Input: part model. Units: mm. Frame: model coordinates. Coordinates: 2 decimals unless noted, no trailing zeros. Loops run counter-clockwise (first coordinate to the right, second up) from the corner with the lowest first, then second, coordinate; pieces in that order, holes last. Notation, with made-up numbers: (34, 70.25) - (45, 70.25) arc R20 ccw to (45, 106.25) - close; hole circle Ø5 at (27.5, -14). An arc over 180 degrees is marked (long way). Write item = value, one per line. Start each with the question number.
from build123d import *

# Parameters (mm, degrees)
F0_W     = 203.2
F0_H     = 38.1
F1_DEPTH = 3.175
F2_W     = 3.175
F2_H     = 4.445
F3_DEPTH = 25.4


# Not quite as in the source:
# - a feature names something its author has since deleted; it is built from what else it names


with BuildPart() as f1:
    # F0 (on Top) → F1 (new body)
    with BuildSketch(Plane.XY):
        with Locations((101.6, -19.05)):
            Rectangle(F0_W, F0_H)
    extrude(amount=F1_DEPTH)

    # F2 (on face) → F3 (cut)
    with BuildSketch(Plane.XY.offset(3.175)):
        with BuildLine():
            Line((0, -9.525), (0, -14.2875))
            ThreePointArc((0, -14.2875), (24.649723028, -4.4760985439), (50.8, 0))
            Line((50.8, 0), (0, 0))
            Line((0, 0), (0, -9.525))
        make_face()
        with Locations((103.1875, -35.8775)):
            Rectangle(F2_W, F2_H)
        with BuildLine():
            ThreePointArc((104.775, -30.48), (103.8450640303, -32.7250640303), (101.6, -33.655))
            Line((101.6, -33.655), (104.775, -33.655))
            Line((104.775, -33.655), (104.775, -30.48))
        make_face()
        with BuildLine():
            Line((104.775, -30.48), (101.6, -30.48))
            Line((101.6, -30.48), (101.6, -33.655))
            ThreePointArc((101.6, -33.655), (103.8450640303, -32.7250640303), (104.775, -30.48))
        make_face()
        with BuildLine():
            Line((101.6, -27.305), (101.6, -30.48))
            Line((101.6, -30.48), (104.775, -30.48))
            ThreePointArc((104.775, -30.48), (103.8450640303, -28.2349359697), (101.6, -27.305))
        make_face()
        with BuildLine():
            Line((98.4250000029, -30.4801362911), (101.6, -30.48))
            Line((101.6, -30.48), (101.6, -27.305))
            ThreePointArc((101.6, -27.305), (99.3548877841, -28.2349841564), (98.4250000029, -30.4801362911))
        make_face()
        with BuildLine():
            Line((101.6, -33.655), (101.6, -30.48))
            Line((101.6, -30.48), (98.4250000029, -30.4801362911))
            ThreePointArc((98.4250000029, -30.4801362911), (99.3549841564, -32.7251122159), (101.6, -33.655))
        make_face()
        with BuildLine():
            ThreePointArc((108.3690122037, -30.48), (106.4969075417, -31.9824905065), (104.775, -33.655))
            Line((104.775, -33.655), (104.775, -38.1))
            Line((104.775, -38.1), (184.15, -38.1))
            Line((184.15, -38.1), (193.675, -26.19375))
            ThreePointArc((193.675, -26.19375), (163.9135585822, -23.6655567526), (134.3847364187, -28.1581971794))
            ThreePointArc((134.3847364187, -28.1581971794), (121.0555708247, -25.7189035938), (108.3690122037, -30.48))
        make_face()
        with BuildLine():
            Line((101.6, -38.1), (101.6, -33.655))
            ThreePointArc((101.6, -33.655), (99.3549841564, -32.7251122159), (98.4250000029, -30.4801362911))
            Line((98.4250000029, -30.4801362911), (39.6036359929, -30.4826612755))
            ThreePointArc((39.6036359929, -30.4826612755), (18.2099329026, -26.2778753266), (0, -14.2875))
            Line((0, -14.2875), (0, -19.05))
            Line((0, -19.05), (0, -38.1))
            Line((0, -38.1), (101.6, -38.1))
        make_face()
        Polygon((203.2, 0), (184.15, 0), (203.2, -14.2875), align=None)
        Polygon((193.675, -26.19375), (184.15, -38.1), (203.2, -38.1), (203.2, -19.05), (203.2, -14.2875), align=None)
        with BuildLine():
            Line((108.3690122037, -30.48), (104.775, -30.48))
            Line((104.775, -30.48), (104.775, -33.655))
            ThreePointArc((104.775, -33.655), (106.4969075417, -31.9824905065), (108.3690122037, -30.48))
        make_face()
        with BuildLine():
            ThreePointArc((127.6218066335, -14.2875), (122.8593066335, -9.525), (118.0968066335, -14.2875))
            Line((118.0968066335, -14.2875), (127.6218066335, -14.2875))
        make_face()
        with BuildLine():
            Line((127.6218066335, -14.2875), (118.0968066335, -14.2875))
            ThreePointArc((118.0968066335, -14.2875), (122.8593066335, -19.05), (127.6218066335, -14.2875))
        make_face()
        with BuildLine():
            Line((176.8343066335, -14.2875), (183.1843066335, -14.2875))
            ThreePointArc((183.1843066335, -14.2875), (180.0093066335, -11.1125), (176.8343066335, -14.2875))
        make_face()
        with BuildLine():
            ThreePointArc((176.8343066335, -14.2875), (180.0093066335, -17.4625), (183.1843066335, -14.2875))
            Line((183.1843066335, -14.2875), (176.8343066335, -14.2875))
        make_face()
        with BuildLine():
            ThreePointArc((155.4030566335, -14.2875), (151.4343066335, -10.31875), (147.4655566335, -14.2875))
            Line((147.4655566335, -14.2875), (155.4030566335, -14.2875))
        make_face()
        with BuildLine():
            Line((155.4030566335, -14.2875), (147.4655566335, -14.2875))
            ThreePointArc((147.4655566335, -14.2875), (151.4343066335, -18.25625), (155.4030566335, -14.2875))
        make_face()
    extrude(amount=-F3_DEPTH, mode=Mode.SUBTRACT)

    # F8: sweep along a path in F5
    with BuildLine(Plane.XY.offset(1.5875)) as f8_path:
        Line((101.6, -30.48), (39.6036359929, -30.4826612755))
        ThreePointArc((39.6036359929, -30.4826612755), (18.2099329026, -26.2778753266), (0, -14.2875))
    # F7 (on offset) → F8 (sweep, cut)
    with BuildSketch(Plane.YZ.offset(101.6)):
        Polygon((-30.48, 3.1877), (-30.48, 1.5875), (-4.1187478461, 6.2357), (-30.48, 6.2357), align=None)
        Polygon((-30.48, 1.5875), (-30.48, 0), (-30.48, -3.0607), (-4.1187478461, -3.0607), align=None)
    sweep(path=f8_path.line, mode=Mode.SUBTRACT)


solid = f1.part
Item 1: Ray query, line 1 (Y direction, x = 123, z = 1.7); line 2 (X direction, y = -12, z = 2.4); line 3 (Y direction, x = 181, z = 0.8). Return the intervals inside material, ascending.
Item 2: Cut plane C-C on x = 90. Return loops of the section in (y, z) (1 decimal).
Item 3: Cut plane B-B on z = 0.5. State how many separate pieces and enclosed holes the cut face has, plus the area to 3 significant figures.
Item 4: Pull-direction query (X, two-part tool) for faces 1 (the flat face through (198.5, -20.16, 1.61)), 2 (the cylindrical face through (24.292, -4.577, 1.61)), 3 (the cylindrical face through (118.317, -15.718, 1.61)); classes: pulls with the +X half, pulls with the -X half, needs draft (parallel to the pull), parting line crosses it, or undercut.
Item 5: Cut plane A-A on x = 46.5. Return loops of the section in (y, z) (1 decimal).
Item 6: Pin query (flat end, axial travel): pin 1 (1 mm diameter, centred on x = 106.5, z = 2, fed in from -Y); pin 2 (1.5 mm diameter, centred on y = -6.5, z = 1, fed in from +X). Return the tip coordinate at first contact, or that it passes through.
Item 7: Cut plane D-D on x = 139. Return loops of the section in (y, z) (3 decimals).
Recorded:
q1.line_1 = -25.62 to -19.05, -9.53 to 0
q1.line_2 = 4.58 to 118.68, 127.04 to 148.19, 154.68 to 177.81, 182.21 to 200.15
q1.line_3 = -24.25 to -17.3, -11.27 to 0
q2.outline = (-30.5, 1.6) - (-21.5, 0) - (0, 0) - (0, 3.2) - (-21.5, 3.2) - close
q3.separate_pieces = 1
q3.enclosed_holes = 3
q3.area = 4,270 mm²
q4.face_1 = pulls with the +X half
q4.face_2 = pulls with the -X half
q4.face_3 = undercut
q5.outline = (-30.5, 1.6) - (-21.5, 0) - (-0.4, 0) - (-0.4, 3.2) - (-21.5, 3.2) - close
q6.pin_1 = -30.48
q6.pin_2 = 193.82
q7.outline = (-26.979, 0) - (0, 0) - (0, 3.175) - (-26.979, 3.175) - close
